Autodesk Inventor part; units mm, degrees
ref_plane "YZ Plane" through (0, 0, 0) normal (1, 0, 0) x (0, 1, 0)
ref_plane "XZ Plane" through (0, 0, 0) normal (0, 1, 0) x (-1, 0, 0)
ref_plane "XY Plane" through (0, 0, 0) normal (0, 0, 1) x (1, 0, 0)
sketch "Эскиз1" plane through (0, 0, 0) normal (0, 1, 0) x (-1, 0, 0)
  line L0 (180.5057, 0) -> (155.5057, 0)
  line L1 (155.5057, 0) -> (155.5057, -46)
  line L2 (155.5057, -46) -> (180.5057, -46)
  line L3 (180.5057, -46) -> (180.5057, 0)
  point P0 (0, 0)
  dimension "d0" = 25
  dimension "d1" = 46
extrude "Выдавливание1" add sketch "Эскиз1" along normal blind 138
fillet "Сопряжение1" radius 2 12 edges at (-155.5057, 69, 0) (-155.5057, 69, -46) (-155.5057, 138, -23) (-155.5057, 0, -23) (-168.0057, 138, 0) (-168.0057, 138, -46) (-180.5057, 138, -23) (-180.5057, 69, 0) (-180.5057, 69, -46) (-180.5057, 0, -23) (-168.0057, 0, 0) (-168.0057, 0, -46)
sketch "Эскиз2" plane through (-180.5057, 2, -2) normal (-1, 0, 0) x (0, 0, 1)
  line L0 (-42.0719, 0.0612) -> (-37.0719, 0.0612)
  line L1 (-37.0719, 0.0612) -> (-37.0719, 3.0612)
  line L2 (-37.0719, 3.0612) -> (-42.0719, 3.0612)
  line L3 (-42.0719, 3.0612) -> (-42.0719, 0.0612)
  line L4 (0, 0) -> (-42, 0)
  line L5 (0, 0) -> (-5, 0)
  line L6 (-5, 0) -> (-5, 3)
  line L7 (-5, 3) -> (0, 3)
  line L8 (0, 3) -> (0, 0)
  point P0 (2, -2)
  dimension "d5" = 5
  dimension "d6" = 3
  dimension "d7" = 5
  dimension "d8" = 3
extrude "Выдавливание2" add sketch "Эскиз2" along normal blind 5
properties part number "Аккумулятор"
Verification items for the finished model (mm, model axes). A direction names the side the tool comes from. Give positions to 0.01 mm unless a question says otherwise; leave off trailing zeros. Write each loop counter-clockwise with the first axis right and the second up, starting at its lowest first coordinate (ties: lowest second). Pieces come first, ordered by that corner, then holes. Notation, with made-up numbers: M 20.5,-10.75 L 56.5,-10.75 A11 cw 56.5,6.25 Z; hole C 86.25,79 d10. An arc over 180 degrees is marked long. Put each result on its own line as item: value. Start each with the question number.
1. Section check B-B (z = -32.5). Record the cut outline in (x, y).
2. Draft check along Z on faces 1 (the face through (-183, 4, -2)), 2 (the face through (-183, 4, -39.072)), 3 (the face through (-183, 2.061, -42)). Enter one of: +Z half, -Z half, draft (parallel to the pull), parting line (faces both ways), or undercut.
3. Section check D-D (z = -40.5). Record the cut outline in (x, y).
4. Section check A-A (x = -181.75). Record the cut outline in (y, z), and give its area (3 significant figures).
5. Section check C-C (y = 56). Record the cut outline in (x, z), and give its area (3 significant figures).
6. Go/stop test with flat-tipped pins: pin 1 Ø1.5 at (x, y) = (-183.5, 4) entering from +Z; pin 2 Ø4 at (x, z) = (-182, -4) entering from +Y; pin 3 Ø5.5 at (x, z) = (-183, -3.5) entering from -Y. Record where each tip stops, or that it passes through.
7. Scan lines: line 1 along X through (y, z) = (7, -29.5); line 2 along Y through (x, z) = (-157.25, -15); line 3 along Y through (x, z) = (-179.5, -21). Record each from-to range of solid material in increasing order. Write a range as [from, to].
8. Set-up check for faces 4 (the face through (-183, 3, -7)), 5 (the face through (-183, 2, -4)), 6 (the face through (-168, 68, -46)), 7 (the face through (-183, 4, -44.072)): record each of +Z, -Z, +X, -X, +Y, -Y from which the full face is reachable in a straight line by a thin tool's end or side.
Answer list:
1. outline: M -180.51,2 A2 ccw -178.51,0 L -157.51,0 A2 ccw -155.51,2 L -155.51,136 A2 ccw -157.51,138 L -178.51,138 A2 ccw -180.51,136 Z
2. face 1: +Z half
2. face 2: undercut
2. face 3: draft
3. outline: M -185.51,2.06 L -180.51,2.06 L -180.51,2 A2 ccw -178.51,0 L -157.51,0 A2 ccw -155.51,2 L -155.51,136 A2 ccw -157.51,138 L -178.51,138 A2 ccw -180.51,136 L -180.51,5.06 L -185.51,5.06 Z
4. outline: M 2,-7 L 5,-7 L 5,-2 L 2,-2 Z; M 2.06,-44.07 L 5.06,-44.07 L 5.06,-39.07 L 2.06,-39.07 Z
4. area: 30.0 mm2
5. outline: M -180.51,-44 A2 ccw -178.51,-46 L -157.51,-46 A2 ccw -155.51,-44 L -155.51,-2 A2 ccw -157.51,0 L -178.51,0 A2 ccw -180.51,-2 Z
5. area: 1,150 mm2
6. pin 1: z = -2
6. pin 2: y = 137.33
6. pin 3: y = 1.02
7. line 1: [-180.51, -155.51]
7. line 2: [0.02, 137.98]
7. line 3: [0.26, 137.74]
8. face 4: -X, +Y, -Y
8. face 5: +Z, -Z, -X, -Y
8. face 6: -Z, +X, -X, +Y, -Y
8. face 7: -Z, -X, +Y, -Y
